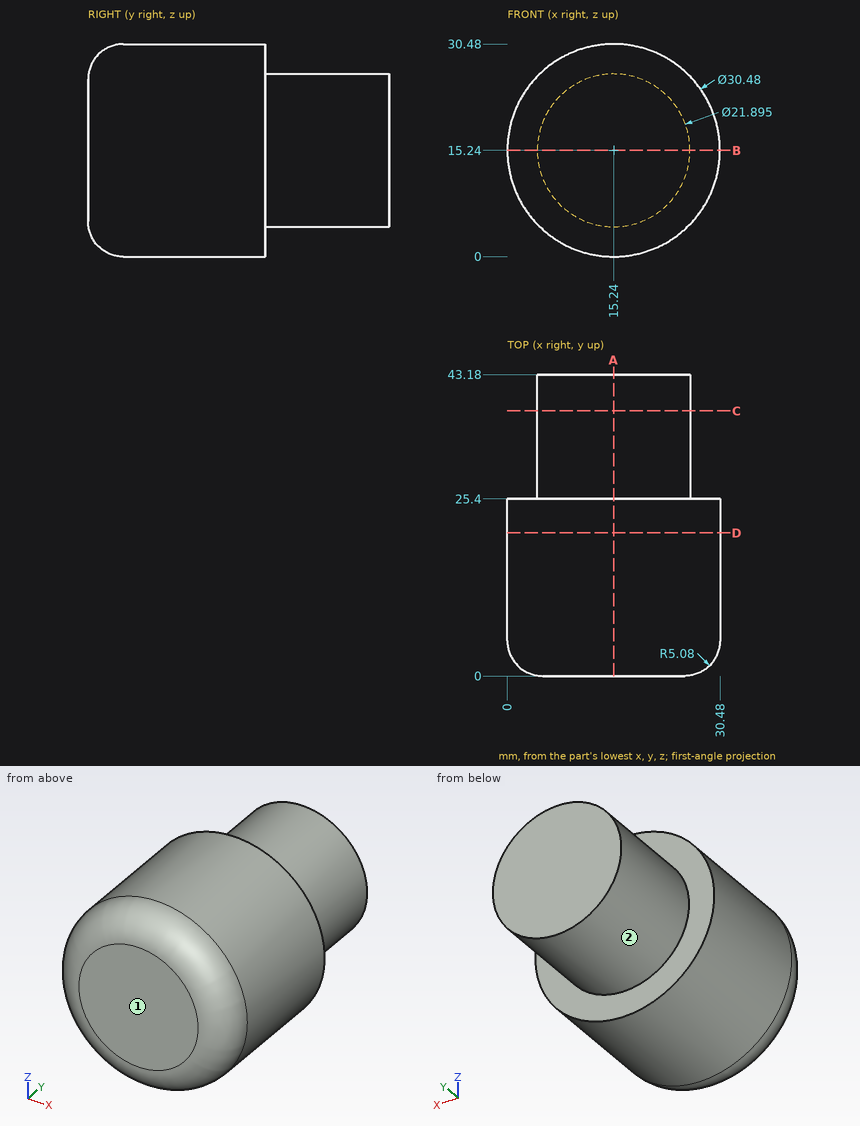
Geometry: see drawing. Coordinates: mm, zero at the bounding-box minimum. A direction names the side the tool comes from. Give positions to 0.01 mm unless a question says otherwise; leave off trailing zeros. Write each loop counter-clockwise with the first axis right and the second up, starting at its lowest first coordinate (ties: lowest second). Pieces come first, ordered by that corner, then holes. Notation, with made-up numbers: M 28,2.5 L 83,2.5 A25 ccw 83,40.5 Z; hole C 58,74.25 d2. An arc over 180 degrees is marked long. Answer in a Markdown table with one row per item. Add a question column.
(1) Section B-B on z = 15.24. Return loops of the section in (x, y), and give its area (3 significant figures).
(2) Reachability of the marked faces 1 and 2 from +Z, -Z, +X, -X, +Y, -Y: full face, straight path, thin tool, end or side. Return the list, or none.
(3) Ray query, line 1 (Y direction, x = 15.5, z = 5); line 2 (X direction, y = 18, z = 15); line 3 (Z direction, x = 11, y = 21). Return the intervals inside material, ascending.
(4) First-contact query: pin 1 (2 mm diameter, centred on y = 22.5, z = 10.5, fed in from -X); pin 2 (12 mm diameter, centred on x = 16.5, z = 3.5, fed in from +Y); pin 3 (6 mm diameter, centred on x = 24, y = 26, fed in from -Z) (1 decimal); pin 4 (3 mm diameter, centred on x = 8, y = 34.5, fed in from -Z). Flat tips, straight axial feed; report the tip coordinate or a pass-through.
(5) Section A-A on x = 15.24. Return loops of the section in (y, z).
(6) Section C-C on y = 38. Return loops of the section in (x, z) (1 decimal).
(7) Section D-D on y = 20.5. Return loops of the section in (x, z), and give its area (3 significant figures).
Result set:
| question | item | result |
|---|---|---|
| 1 | outline | M 0,5.08 A5.08 ccw 5.08,0 L 25.4,0 A5.08 ccw 30.48,5.08 L 30.48,25.4 L 26.19,25.4 L 26.19,43.18 L 4.29,43.18 L 4.29,25.4 L 0,25.4 Z |
| 1 | area | 1,150 mm^2 |
| 2 | face 1 | +Z, -Z, +X, -X, -Y |
| 2 | face 2 | +Y |
| 3 | line 1 | y = 0 to 43.18 |
| 3 | line 2 | x = 0 to 30.48 |
| 3 | line 3 | z = 0.6 to 29.88 |
| 4 | pin 1 | stops at x = 0.47 |
| 4 | pin 2 | stops at y = 43.18 |
| 4 | pin 3 | stops at z = 1.2 |
| 4 | pin 4 | stops at z = 5.92 |
| 5 | outline | M 0,5.08 A5.08 ccw 5.08,0 L 25.4,0 L 25.4,4.29 L 43.18,4.29 L 43.18,26.19 L 25.4,26.19 L 25.4,30.48 L 5.08,30.48 A5.08 ccw 0,25.4 Z |
| 6 | outline | C 15.2,15.2 d21.9 |
| 7 | outline | C 15.24,15.24 d30.48 |
| 7 | area | 730 mm^2 |
